Geometry: final body of the model. Coordinates: model frame, mm. Face numbers are marked on the shaded views. A direction names the side the tool comes from. Give positions to 0.01 mm unless a question says otherwise; leave off trailing zeros. Write each loop counter-clockwise with the first axis right and the second up, starting at its lowest first coordinate (ties: lowest second). Pieces come first, ordered by that corner, then holes. Notation, with made-up numbers: (79, 10) -> (125, 10) arc R15 ccw to (125, 26) -> close; hole circle Ø1 at (41.5, 10.25). An arc over 180 degrees is marked (long way). Answer as a JSON object with one key per item and string values.
from build123d import *

# Parameters (mm, degrees)
SKETCH058_R     = 30
PAD035_DEPTH    = 7.25
SKETCH067_R     = 25
POCKET016_DEPTH = 5
SKETCH068_R     = 3
PAD040_DEPTH    = 4
SKETCH069_R     = 1
POCKET017_DEPTH = 4


with BuildPart() as part:
    # Sketch058 → Pad035 (new body)
    with BuildSketch(Plane.YZ):
        with Locations((50, 14)):
            Circle(SKETCH058_R)
    extrude(amount=PAD035_DEPTH)

    # Sketch067 (on Face3 of Pad035) → Pocket016 (cut)
    with BuildSketch(Plane.YZ.offset(7.25)):
        with Locations((50, 14)):
            Circle(SKETCH067_R)
    extrude(amount=-POCKET016_DEPTH, mode=Mode.SUBTRACT)

    # Sketch068 (on Face5 of Pocket016) → Pad040 (join)
    with BuildSketch(Plane.YZ.offset(2.25)):
        with Locations((50, 14)):
            Circle(SKETCH068_R)
    extrude(amount=PAD040_DEPTH)

    # Sketch069 (on Face7 of Pad040) → Pocket017 (cut)
    with BuildSketch(Plane.YZ.offset(6.25)):
        with Locations((50, 14)):
            Circle(SKETCH069_R)
    extrude(amount=-POCKET017_DEPTH, mode=Mode.SUBTRACT)


solid = part.part
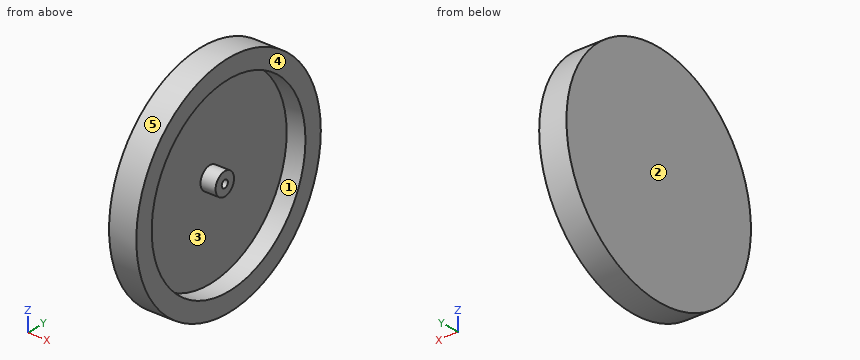
Q1. Set-up query: the marked faces 1 and 2. Return all of +Z, -Z, +X, -X, +Y, -Y with unobstructed straight access to the full face (end or side cutting, diameter ignored); none if empty.
Values:
{"face 1": "+X", "face 2": "+Z, -Z, -X, +Y, -Y"}
Q2. Cut plane A-A (x = 4.25). Return the cut outline in (y, z), and give its area (3 significant figures).
Values:
{"outline": "circle Ø60 at (50, 14); circle Ø6 at (50, 14); hole circle Ø50 at (50, 14); hole circle Ø2 at (50, 14)", "area": "889 mm²"}
Q3. Cut plane D-D (z = 14). Return the cut outline in (x, y).
Values:
{"outline": "(0, 20) -> (7.25, 20) -> (7.25, 25) -> (2.25, 25) -> (2.25, 47) -> (6.25, 47) -> (6.25, 49) -> (2.25, 49) -> (2.25, 51) -> (6.25, 51) -> (6.25, 53) -> (2.25, 53) -> (2.25, 75) -> (7.25, 75) -> (7.25, 80) -> (0, 80) -> close"}
Q4. Cut plane C-C (y = 50). Return the cut outline in (x, z), and give its area (3 significant figures).
Values:
{"outline": "(0, -16) -> (7.25, -16) -> (7.25, -11) -> (2.25, -11) -> (2.25, 11) -> (6.25, 11) -> (6.25, 13) -> (2.25, 13) -> (2.25, 15) -> (6.25, 15) -> (6.25, 17) -> (2.25, 17) -> (2.25, 39) -> (7.25, 39) -> (7.25, 44) -> (0, 44) -> close", "area": "201 mm²"}
Q5. First-contact query: P1, Ø1.6, axis at y = 50, z = 14, coming from the +X side; P2, Ø1, axis at x = 6.5, z = 6.5, coming from the -Y side; P3, Ø1.5, axis at x = 4.5, y = 73.5, coming from the +Z side; P4, Ø12, axis at y = 67.5, z = 29, coming from the -X side. Flat tips, straight axial feed; report the tip coordinate or a pass-through.
Values:
{"P1": "x = 2.25", "P2": "y = 20.83", "P3": "z = 33.56", "P4": "x = 0"}
Q6. Material intervals for L1, parallel to Z at x = 3.65, y = 50; L2, parallel to Y at x = 2.5, z = 12; L3, parallel to X at y = 70, z = 8, sorted ascending. Write a range as from..to.
Values:
{"L1": "-16..-11, 11..13, 15..17, 39..44", "L2": "20.07..25.08, 47.76..52.24, 74.92..79.93", "L3": "0..2.25"}
Q7. Mould query, pull axis Y, two halves, no side actions, for the marked faces 3, 4 and 5. Classes: pulls with the +Y half, pulls with the -Y half, needs draft (parallel to the pull), parting line crosses it, or undercut.
Values:
{"face 3": "undercut", "face 4": "needs draft", "face 5": "parting line crosses it"}
Q8. Cut plane B-B (z = 0.5). Return the cut outline in (x, y), and give its area (3 significant figures).
Values:
{"outline": "(0, 23.21) -> (7.25, 23.21) -> (7.25, 28.96) -> (2.25, 28.96) -> (2.25, 71.04) -> (7.25, 71.04) -> (7.25, 76.79) -> (0, 76.79) -> close", "area": "178 mm²"}
